```python
from build123d import *

# Parameters (mm, degrees)
SKETCH_2_R      = 1.5
SKETCH_2_R_2    = 1
EXTRUDE_1_DEPTH = 0.5
SKETCH_1_R      = 1.5
SKETCH_1_R_2    = 1
EXTRUDE_2_DEPTH = 0.5
SKETCH_4_W      = 17
SKETCH_4_H      = 11
EXTRUDE_4_DEPTH = 0.5


with BuildPart() as part:
    # Sketch 2 → Extrude 1 (new body)
    with BuildSketch(Plane.XY.offset(10)):
        with BuildLine():
            Line((15, 5), (-15, 5))
            Line((-15, 5), (-15, -5))
            Line((-15, -5), (15, -5))
            ThreePointArc((15, -5), (20, 0), (15, 5))
        make_face()
        with Locations((15, 0)):
            Circle(SKETCH_2_R, mode=Mode.SUBTRACT)
        with Locations((11, -3)):
            Circle(SKETCH_2_R_2, mode=Mode.SUBTRACT)
        with Locations((11, 3)):
            Circle(SKETCH_2_R_2, mode=Mode.SUBTRACT)
        with Locations((2, 0)):
            Circle(SKETCH_2_R_2, mode=Mode.SUBTRACT)
        with Locations((-4, 0)):
            Circle(SKETCH_2_R_2, mode=Mode.SUBTRACT)
        with Locations((-10, 0.253438211)):
            Circle(SKETCH_2_R_2, mode=Mode.SUBTRACT)
    extrude(amount=EXTRUDE_1_DEPTH)



with BuildPart() as body_2:
    # Sketch 1 → Extrude 2 (new body)
    with BuildSketch(Plane.XY):
        with BuildLine():
            Line((-15, 5), (15, 5))
            ThreePointArc((15, 5), (20, 0), (15, -5))
            Line((15, -5), (-15, -5))
            Line((-15, -5), (-15, 5))
        make_face()
        with Locations((15, 0)):
            Circle(SKETCH_1_R, mode=Mode.SUBTRACT)
        with Locations((-10, 0.253438211)):
            Circle(SKETCH_1_R_2, mode=Mode.SUBTRACT)
        with Locations((-4, 0)):
            Circle(SKETCH_1_R_2, mode=Mode.SUBTRACT)
        with Locations((2, 0)):
            Circle(SKETCH_1_R_2, mode=Mode.SUBTRACT)
        with Locations((11, 3)):
            Circle(SKETCH_1_R_2, mode=Mode.SUBTRACT)
        with Locations((11, -3)):
            Circle(SKETCH_1_R_2, mode=Mode.SUBTRACT)
    extrude(amount=-EXTRUDE_2_DEPTH)


with BuildPart() as part_1:
    add(part.part)

    add(body_2.part)  # Extrude 4 merges body 2
    # Sketch 4 → Extrude 4 (add)
    with BuildSketch(Plane(origin=(0, -5, 0), x_dir=(1, 0, 0), z_dir=(0, 1, 0))):
        with Locations((-6.5, -5)):
            Rectangle(SKETCH_4_W, SKETCH_4_H)
    extrude(amount=-EXTRUDE_4_DEPTH)


solid = part_1.part
```
Part model, mm, in its own coordinate system. A direction names the side the tool comes from. Round coordinates to 2 decimals unless told otherwise and drop trailing zeros. Write each loop counter-clockwise with the first axis right and the second up, starting at its lowest first coordinate (ties: lowest second). Pieces come first, ordered by that corner, then holes. Notation, with made-up numbers: M 41,79.5 L 58,79.5 A23 cw 58,111.5 Z; hole C 74,9 d1. An arc over 180 degrees is marked long. One line per question, with ' | ' between items.
(1) Probe line 1 along Y through (x, z) = (-4, -0.05); line 2 along Y through (x, z) = (-10, -0.1); line 3 along Z through (x, y) = (3, -2.5). List the from-to ranges inside material, lowest first.
Answer key:
line 1: y = -5.5 to -1, 1 to 5 | line 2: y = -5.5 to -0.75, 1.25 to 5 | line 3: z = -0.5 to 0, 10 to 10.5
(2) Saw through at B-B on y = 3. Write the cut outline in (x, z).
Answer key:
outline: M -15,-0.5 L 10,-0.5 L 10,0 L -15,0 Z; M -15,10 L 10,10 L 10,10.5 L -15,10.5 Z; M 12,-0.5 L 19,-0.5 L 19,0 L 12,0 Z; M 12,10 L 19,10 L 19,10.5 L 12,10.5 Z
(3) 3-axis set-ups, long thin cutter, end or side, ignore diameter. For faces 1 (the face through (20, 0.1, -0.2)), 2 (the face through (-7, -5, 5)): which of +Z, -Z, +X, -X, +Y, -Y reach the whole face in a straight line?
Answer key:
face 1: +Z, -Z, +X | face 2: +X, -X, +Y
(4) Two-plate mould, pull along Z, no slides. Class faces 3 (the face through (2.3, 1.2, 10)), 4 (the face through (2.3, -1.3, 10.5)), 5 (the face through (10.263, 3.676, 10.246)): released by +Z, released by -Z, zero draft, split by the parting line, or undercut.
Answer key:
face 3: undercut | face 4: released by +Z | face 5: zero draft
(5) Saw through at A-A on x = 11. Write the cut outline in (y, z).
Answer key:
outline: M -5,-0.5 L -4,-0.5 L -4,0 L -5,0 Z; M -5,10 L -4,10 L -4,10.5 L -5,10.5 Z; M -2,-0.5 L 2,-0.5 L 2,0 L -2,0 Z; M -2,10 L 2,10 L 2,10.5 L -2,10.5 Z; M 4,-0.5 L 5,-0.5 L 5,0 L 4,0 Z; M 4,10 L 5,10 L 5,10.5 L 4,10.5 Z
(6) Saw through at D-D on y = -4.5. Write the cut outline in (x, z).
Answer key:
outline: M -15,-0.5 L 17.18,-0.5 L 17.18,0 L -15,0 Z; M -15,10 L 17.18,10 L 17.18,10.5 L -15,10.5 Z
(7) Saw through at C-C on x = -10. Write the cut outline in (y, z).
Answer key:
outline: M -5.5,-0.5 L -0.75,-0.5 L -0.75,0 L -5,0 L -5,10 L -0.75,10 L -0.75,10.5 L -5.5,10.5 Z; M 1.25,-0.5 L 5,-0.5 L 5,0 L 1.25,0 Z; M 1.25,10 L 5,10 L 5,10.5 L 1.25,10.5 Z
